Autodesk Fusion 360 part; units mm, degrees
sketch "Sketch1" plane through (0, 0, 0) normal (0, 0, 1) x (1, 0, 0)
  line L0 (0, 0) -> (50, 0)
  line L1 (50, 0) -> (50, 10)
  line L2 (50, 10) -> (0, 10)
  line L3 (0, 10) -> (0, 0)
  line L4 (50, 0) -> (40, 0)
  line L5 (40, 0) -> (40, -18)
  line L6 (40, -18) -> (50, -18)
  line L7 (50, -18) -> (50, 0)
  circle A0 centre (5, 5.625) radius 1.8
  circle A1 centre (35, 5.625) radius 1.8
  circle A2 centre (45, 5.625) radius 2.3
  circle A3 centre (45, -12.375) radius 2.3
  circle A4 centre (10, 5.625) radius 1.8
  line L8 (5.039, 3.8254) -> (10, 3.8254)
  line L9 (10, 7.425) -> (5, 7.425)
  dimension "d1" = 50
  dimension "d2" = 10
  dimension "d3" = 10
  dimension "d4" = 18
  dimension "d5" = 3.6
  dimension "d6" = 3.6
  dimension "d7" = 5
  dimension "d8" = 30
  dimension "d9" = 4.6
  dimension "d10" = 10
  dimension "d11" = 4.6
  dimension "d12" = 18
  dimension "d20" = 3.6
  dimension "d21" = 5.625
  dimension "d22" = 5
extrude "Extrude1" add sketch "Sketch1" along normal blind 8
fillet "Fillet1" radius 3 5 edges at (40, -18, 4) (50, -18, 4) (0, 0, 4) (50, 10, 4) (0, 10, 4)
fillet "Fillet2" radius 18 1 edges at (40, 0, 4)
chamfer "Chamfer1" [suppressed]
equation "d4 = d12"
equation "d6 = d5"
equation "d9 = d11"
equation "d20 = d5"
equation "d21 = 9 / 16 * d2"
Part model, mm, in its own coordinate system. A direction names the side the tool comes from. Give positions to 0.01 mm unless a question says otherwise; leave off trailing zeros. Loops run counter-clockwise (first coordinate to the right, second up) from the corner with the lowest first, then second, coordinate; pieces in that order, holes last.
(1) Band-saw the part on C-C (y = 4.5). Write the cut outline in (x, z).
Return value:
outline: (0, 0) - (3.59, 0) - (3.59, 8) - (0, 8) - close; (11.41, 0) - (33.59, 0) - (33.59, 8) - (11.41, 8) - close; (36.41, 0) - (42.99, 0) - (42.99, 8) - (36.41, 8) - close; (47.01, 0) - (50, 0) - (50, 8) - (47.01, 8) - close
(2) Pull direction Y, two halves, no side cores. Call faces 4 (the flat face through (30, 2, 8)), 5 (the cylindrical face through (0.86, 0.9, 4.06)), 6 (the cylindrical face through (11.8, 5.7, 3.9)): pulls with the +Y half, pulls with the -Y half, needs draft (parallel to the pull), parting line crosses it, or undercut.
Return value:
face 4: needs draft
face 5: pulls with the -Y half
face 6: undercut
(3) Band-saw the part on D-D (z = 5). Count the separate pieces of the cut face and the enclosed holes in it, and give its area (3 significant figures).
Return value:
separate pieces: 1
enclosed holes: 4
area: 665 mm2
(4) Pin check, flat tips, straight feed: pin 1 (8 mm diameter, centred on x = 9.5, y = -0.5, fed in from -Z); pin 2 (3 mm diameter, centred on x = 35, y = 5.625, fed in from -Z); pin 3 (2.5 mm diameter, centred on x = 8, z = 3, fed in from -Y). Stop position of each tip, or through.
Return value:
pin 1: stops at z = 0
pin 2: passes through
pin 3: stops at y = 0
(5) Band-saw the part on A-A (x = 6). Write the cut outline in (y, z) (3 decimals).
Return value:
outline: (0, 0) - (3.825, 0) - (3.825, 8) - (0, 8) - close; (7.425, 0) - (10, 0) - (10, 8) - (7.425, 8) - close
(6) Drill centre lines: line 1 along Y through (x, z) = (45, 6) (3 decimals); line 2 along X through (y, z) = (7.25, 6.25); line 3 along Y through (x, z) = (4, 4.5). Where is each one in solid material? Low to high.
Return value:
line 1: y = -18 to -14.675, -10.075 to 3.325, 7.925 to 10
line 2: x = 0.01 to 4.23, 10.77 to 34.23, 35.77 to 43.37, 46.63 to 49.99
line 3: y = 0 to 4.13, 7.12 to 10
(7) 3-axis set-ups, long thin cutter, end or side, ignore diameter. For faces 1 (the flat face through (12, 0, 4)), 2 (the cylindrical face through (49.14, 9.1, 4.06)), 3 (the cylindrical face through (3.2, 5.6, 3.9)): which of +Z, -Z, +X, -X, +Y, -Y reach the whole face in a straight line?
Return value:
face 1: +Z, -Z, -X, -Y
face 2: +Z, -Z, +X, +Y
face 3: +Z, -Z
(8) Band-saw the part on B-B (x = 45). Write the cut outline in (y, z) (3 decimals).
Return value:
outline: (-18, 0) - (-14.675, 0) - (-14.675, 8) - (-18, 8) - close; (-10.075, 0) - (3.325, 0) - (3.325, 8) - (-10.075, 8) - close; (7.925, 0) - (10, 0) - (10, 8) - (7.925, 8) - close
